from build123d import *

# Parameters (mm, degrees)
SKETCH1_R           = 5.675
BOSS_EXTRUDE1_DEPTH = 76.6
BOSS_EXTRUDE2_DEPTH = 2
SKETCH3_R           = 4.83
CUT_EXTRUDE1_DEPTH  = 80.545861523
BOSS_EXTRUDE3_START = -1
SKETCH4_R           = 4.83
SKETCH4_R_2         = 1.71
BOSS_EXTRUDE3_DEPTH = 1
SKETCH5_R           = 4.83
SKETCH5_R_2         = 2.4
BOSS_EXTRUDE4_DEPTH = 1


with BuildPart() as part:
    # Sketch1 → Boss-Extrude1 (new body)
    with BuildSketch(Plane(origin=(0, 0, 0), x_dir=(0, 0, -1), z_dir=(1, 0, 0))):
        Circle(SKETCH1_R)
    extrude(amount=-BOSS_EXTRUDE1_DEPTH)

    # Sketch2 → Boss-Extrude2 (add)
    with BuildSketch(Plane.ZY.offset(76.6)):
        with BuildLine():
            Line((-10.125, -2.7), (-10.125, 2.7))
            ThreePointArc((-10.125, 2.7), (0, 6.860645772), (10.125, 2.7))
            Line((10.125, 2.7), (10.125, -2.7))
            ThreePointArc((10.125, -2.7), (0, -6.860645772), (-10.125, -2.7))
        make_face()
    extrude(amount=BOSS_EXTRUDE2_DEPTH)

    # Sketch3 → Cut-Extrude1 (cut, through all)
    with BuildSketch(Plane(origin=(0, 0, 0), x_dir=(0, 0, -1), z_dir=(1, 0, 0))):
        Circle(SKETCH3_R)
    extrude(amount=-CUT_EXTRUDE1_DEPTH, mode=Mode.SUBTRACT)

    # Sketch4 → Boss-Extrude3 (add)
    with BuildSketch(Plane.ZY.offset(60).offset(BOSS_EXTRUDE3_START)):
        with Locations(Location((0, 0, 0), (0, 0, 180))):
            Circle(SKETCH4_R)
        Circle(SKETCH4_R_2, mode=Mode.SUBTRACT)
    extrude(amount=BOSS_EXTRUDE3_DEPTH)

    # Sketch5 → Boss-Extrude4 (add)
    with BuildSketch(Plane(origin=(-5.4, 0, 0), x_dir=(0, 0, -1), z_dir=(1, 0, 0))):
        Circle(SKETCH5_R)
        Circle(SKETCH5_R_2, mode=Mode.SUBTRACT)
    extrude(amount=-BOSS_EXTRUDE4_DEPTH)


solid = part.part
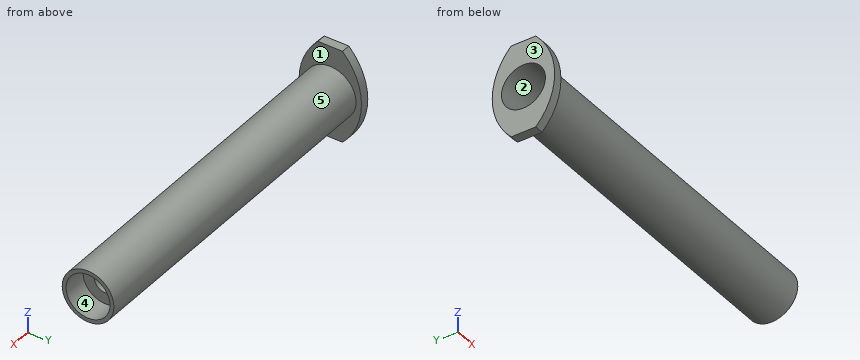
Here's how the part is built. I have some questions about the finished solid (model axes, mm). Face numbers are marked on the shaded views. A direction names the side the tool comes from. Round coordinates to 2 decimals unless told otherwise and drop trailing zeros. Order: outer loops, then holes, each group sorted by start corner. A loop starts at its lowest first (then second) coordinate and runs counter-clockwise, first axis right, second up. Notation, with made-up numbers: M -34.5,60.5 L -2.5,60.5 A28 cw -2.5,80.5 Z; hole C -4,12 d7. An arc over 180 degrees is marked long. One line per question, with ' | ' between items.
1) Imagine slicing it at B-B, the plane y = 0. Write out the boundary of the cut face in (x, z) (3 decimals).
Checked values:
outline: M -78.6,-10.125 L -76.6,-10.125 L -76.6,-5.675 L 0,-5.675 L 0,-4.83 L -5.4,-4.83 L -5.4,-2.4 L -6.4,-2.4 L -6.4,-4.83 L -59,-4.83 L -59,-1.71 L -60,-1.71 L -60,-4.83 L -78.6,-4.83 Z; M -78.6,4.83 L -60,4.83 L -60,1.71 L -59,1.71 L -59,4.83 L -6.4,4.83 L -6.4,2.4 L -5.4,2.4 L -5.4,4.83 L 0,4.83 L 0,5.675 L -76.6,5.675 L -76.6,10.125 L -78.6,10.125 Z
2) I'm going to push flat-ended pins straight in: pin 1 Ø2 at (y, z) = (-3.5, 0) entering from -X; pin 2 Ø3 at (y, z) = (0, 0) entering from -X; pin 3 Ø7.5 at (y, z) = (0.5, -1.5) entering from +X; pin 4 Ø1 at (x, y) = (-57, -5) entering from +Z. Where does each tip first touch, or does it pass through?
Checked values:
pin 1: stops at x = -60 | pin 2: passes through | pin 3: stops at x = 0 | pin 4: stops at z = 3.46
3) Imagine slicing it at C-C, the plane y = 4. Write out the boundary of the cut face in (x, z).
Checked values:
outline: M -78.6,-8.61 L -76.6,-8.61 L -76.6,-4.03 L 0,-4.03 L 0,-2.71 L -5.4,-2.71 L -5.4,2.71 L 0,2.71 L 0,4.03 L -76.6,4.03 L -76.6,8.61 L -78.6,8.61 L -78.6,2.71 L -60,2.71 L -60,-2.71 L -78.6,-2.71 Z; hole M -59,-2.71 L -6.4,-2.71 L -6.4,2.71 L -59,2.71 Z
4) Imagine slicing it at A-A, the plane z = 0. Write out the boundary of the cut face in (x, y) (3 decimals), plus the area to 3 significant figures.
Checked values:
outline: M -78.6,-6.861 L -76.6,-6.861 L -76.6,-5.675 L 0,-5.675 L 0,-4.83 L -5.4,-4.83 L -5.4,-2.4 L -6.4,-2.4 L -6.4,-4.83 L -59,-4.83 L -59,-1.71 L -60,-1.71 L -60,-4.83 L -78.6,-4.83 Z; M -78.6,4.83 L -60,4.83 L -60,1.71 L -59,1.71 L -59,4.83 L -6.4,4.83 L -6.4,2.4 L -5.4,2.4 L -5.4,4.83 L 0,4.83 L 0,5.675 L -76.6,5.675 L -76.6,6.861 L -78.6,6.861 Z | area: 149 mm²
5) I need wall thicknesses on line 1 (Z direction, x = -34, y = -0.25); line 2 (Y direction, x = -59.55, z = 0) (3 decimals); line 3 (Y direction, x = -1.95, z = 0) (3 decimals). Which ranges of each line are inside material? Lowest first, please.
Checked values:
line 1: z = -5.67 to -4.82, 4.82 to 5.67 | line 2: y = -5.675 to -1.71, 1.71 to 5.675 | line 3: y = -5.675 to -4.83, 4.83 to 5.675
6) On a 3-axis mill with a long thin cutter (end or side, diameter ignored), from which of +Z, -Z, +X, -X, +Y, -Y can I reach the whole of each face in a straight line? I mean the marked faces 1 and 2. Say none if no direction works.
Checked values:
face 1: +X | face 2: -X
7) Imagine slicing it at D-D, the plane x = -46. Write out the boundary of the cut face in (y, z) (3 decimals), plus the area to 3 significant figures.
Checked values:
outline: C 0,0 d11.35; hole C 0,0 d9.66 | area: 27.9 mm²
8) We'd pull the mould along Z, two halves only. Please class the marked faces 3, 4 and 5: released by +Z, released by -Z, zero draft, split by the parting line, or undercut.
Checked values:
face 3: zero draft | face 4: undercut | face 5: split by the parting line
